```python
from build123d import *

# Parameters (mm, degrees)
F1_DEPTH = 6.35
F2_R     = 5.08


with BuildPart() as f1:
    # F0 (on Front) → F1 (new body)
    with BuildSketch(Plane.XZ):
        with BuildLine():
            ThreePointArc((18.9777384701, -1.657691938), (19.0319260436, -0.8296330951), (19.05, 0))
            ThreePointArc((19.05, 0), (19.0258577103, 0.9587692038), (18.9534920329, 1.9151082886))
            ThreePointArc((18.9534920329, 1.9151082886), (0, 19.05), (-18.9534920329, 1.9151082886))
            ThreePointArc((-18.9534920329, 1.9151082886), (-19.0495613397, 0.1292778667), (-18.9777384701, -1.657691938))
            ThreePointArc((-18.9777384701, -1.657691938), (0, -19.05), (18.9777384701, -1.657691938))
        make_face()
        with BuildLine():
            ThreePointArc((-18.9534920329, 1.9151082886), (0, 19.05), (18.9534920329, 1.9151082886))
            Line((18.9534920329, 1.9151082886), (12.6356613553, 64.4415743522))
            ThreePointArc((12.6356613553, 64.4415743522), (12.6839051402, 63.8040149624), (12.7, 63.1648354932))
            ThreePointArc((12.7, 63.1648354932), (-0.6391794692, 50.480930353), (-12.6356613553, 64.4415743522))
            Line((-12.6356613553, 64.4415743522), (-18.9534920329, 1.9151082886))
        make_face()
        with BuildLine():
            Line((13.8028917705, -60.9008390119), (18.9777384701, -1.657691938))
            ThreePointArc((18.9777384701, -1.657691938), (0, -19.05), (-18.9777384701, -1.657691938))
            Line((-18.9777384701, -1.657691938), (-12.6518256467, -74.0785781066))
            ThreePointArc((-12.6518256467, -74.0785781066), (-9.1612035414, -64.1778632049), (0.5892201669, -60.2871260312))
            Line((0.5892201669, -60.2871260312), (13.8028917705, -60.9008390119))
        make_face()
        with BuildLine():
            ThreePointArc((12.7, 63.1648354932), (12.6839051402, 63.8040149624), (12.6356613553, 64.4415743522))
            ThreePointArc((12.6356613553, 64.4415743522), (0, 75.8648354932), (-12.6356613553, 64.4415743522))
            ThreePointArc((-12.6356613553, 64.4415743522), (-0.6391794692, 50.480930353), (12.7, 63.1648354932))
        make_face()
        with BuildLine():
            Line((68.8755877414, -63.4587070604), (13.8028917705, -60.9008390119))
            Line((13.8028917705, -60.9008390119), (12.6518256467, -74.0785781066))
            ThreePointArc((12.6518256467, -74.0785781066), (8.795586943, -82.1346536894), (0.5892201669, -85.6597742647))
            Line((0.5892201669, -85.6597742647), (68.8755877414, -82.4881932355))
            ThreePointArc((68.8755877414, -82.4881932355), (58.9086726163, -72.973450148), (68.8755877414, -63.4587070604))
        make_face()
        with BuildLine():
            Line((12.6518256467, -74.0785781066), (13.8028917705, -60.9008390119))
            Line((13.8028917705, -60.9008390119), (0.5892201669, -60.2871260312))
            ThreePointArc((0.5892201669, -60.2871260312), (9.1862151107, -64.2039888224), (12.7, -72.973450148))
            ThreePointArc((12.7, -72.973450148), (12.6879506957, -73.526538878), (12.6518256467, -74.0785781066))
        make_face()
        with BuildLine():
            ThreePointArc((0.5892201669, -60.2871260312), (-9.1612035414, -64.1778632049), (-12.6518256467, -74.0785781066))
            ThreePointArc((-12.6518256467, -74.0785781066), (-8.3610788092, -82.5328623237), (0.5892201669, -85.6597742647))
            ThreePointArc((0.5892201669, -85.6597742647), (8.795586943, -82.1346536894), (12.6518256467, -74.0785781066))
            ThreePointArc((12.6518256467, -74.0785781066), (12.6879506957, -73.526538878), (12.7, -72.973450148))
            ThreePointArc((12.7, -72.973450148), (9.1862151107, -64.2039888224), (0.5892201669, -60.2871260312))
        make_face()
        with BuildLine():
            ThreePointArc((77.9586726163, -72.973450148), (75.3233339493, -66.3963541538), (68.8755877414, -63.4587070604))
            ThreePointArc((68.8755877414, -63.4587070604), (58.9086726163, -72.973450148), (68.8755877414, -82.4881932355))
            ThreePointArc((68.8755877414, -82.4881932355), (75.3233339493, -79.5505461421), (77.9586726163, -72.973450148))
        make_face()
    extrude(amount=F1_DEPTH)

    # F2
    f2_edges = [f1.edges().sort_by_distance(p)[0] for p in [
        (13.802892, -3.175, -60.900839),
    ]]
    fillet(f2_edges, radius=F2_R)


solid = f1.part
```
For this review, take the finished solid that the model builds, in its own axes (mm). Round coordinates to 2 decimals unless told otherwise and drop trailing zeros. Loops run counter-clockwise (first coordinate to the right, second up) from the corner with the lowest first, then second, coordinate; pieces in that order, holes last.
(1) Mouldability with a two-part tool opening along Z and no side actions: class faces 1 (the cylindrical face through (15.54, -3.22, -59.46)), 2 (the flat face through (16.588, -3.131, -29.022)), 3 (the flat face through (7, -6.35, -22)), 4 (the flat face through (15.84, -3.13, 32.74)) as released by +Z, released by -Z, zero draft, split by the parting line, or undercut.
Returned:
face 1: undercut
face 2: undercut
face 3: zero draft
face 4: released by +Z
(2) We need section C-C (z = -58). Give the boundary of the cut face in (x, y).
Returned:
outline: (-14.06, -6.35) - (14.62, -6.35) - (14.62, 0) - (-14.06, 0) - close
(3) Clearance check with flat-ended pins moving along their axes: P1, Ø3, axis at x = 51.5, y = -1.5, coming from the -Z side; P2, Ø2, axis at x = 32, y = -4.5, coming from the -Z side. State where each tip first meets the part, or that it passes through.
Returned:
P1: stops at z = -83.36
P2: stops at z = -84.25
(4) We need section B-B (x = 24). Give the boundary of the cut face in (y, z).
Returned:
outline: (-6.35, -84.57) - (0, -84.57) - (0, -61.37) - (-6.35, -61.37) - close
(5) Wall thickness on line 1 along X through (y, z) = (-2.5, 0); line 2 along X through (y, z) = (-4.5, -10.5); line 3 along Z through (x, y) = (62, -4.25): over which ranges is each line inside the solid? List them lowest first.
Returned:
line 1: x = -19.05 to 19.05
line 2: x = -18.21 to 18.21
line 3: z = -82.81 to -63.14
